from build123d import *

# Parameters (mm, degrees)
SKETCH1_W                  = 210
SKETCH1_H                  = 20
SKETCH2_R                  = 170.296824317
BOSS_EXTRUDE1_DEPTH        = 170
BOSS_EXTRUDE1_TAPER        = 16.950103548
F_8_4_8_4_DIAMETER_HOLE1_D = 8.4
F_8_4_8_4_DIAMETER_HOLE2_D = 8.4
FILLET1_R                  = 2
FILLET2_R                  = 5
FILLET3_R                  = 22
FILLET4_R                  = 25


with BuildPart() as part:
    # Sketch1 → Revolve1 (revolve)
    with BuildSketch(Plane.XZ, mode=Mode.PRIVATE) as revolve1_sk:
        with Locations((105, 10)):
            Rectangle(SKETCH1_W, SKETCH1_H)
    revolve(revolve1_sk.sketch.rotate(Axis((0, 0, 20), (0, 0, -1)), 180), axis=Axis((0, 0, 20), (0, 0, -1)))

    # Sketch2 → Boss-Extrude1 (add)
    with BuildSketch(Plane.XY.offset(20)):
        Circle(SKETCH2_R)
    extrude(amount=BOSS_EXTRUDE1_DEPTH, taper=BOSS_EXTRUDE1_TAPER)

    # Sketch3 → Cut-Revolve1 (revolve, cut)
    with BuildSketch(Plane(origin=(0, 0, 0), x_dir=(1, 0, 0), z_dir=(0, 1, 0))):
        Polygon((155.484121585, 0), (0, 0), (0, -190), (50, -190), (50, -170), (103.671746464, -170), align=None)
    revolve(axis=Axis((0, 0, 0), (0, 0, 1)), mode=Mode.SUBTRACT)

    # Ø8.4 (8.4) Diameter Hole1 (through all)
    with Locations(Plane.XY.offset(20)):
        with Locations((0, 195), (97.5, 168.874953738), (168.874953738, 97.5), (195, 0), (168.874953738, -97.5), (97.5, -168.874953738), (0, -195), (-97.5, -168.874953738), (-168.874953738, -97.5), (-195, 0), (-168.874953738, 97.5), (-97.5, 168.874953738)):
            Hole(F_8_4_8_4_DIAMETER_HOLE1_D / 2)

    # Ø8.4 (8.4) Diameter Hole2 (through all)
    with Locations(Plane(origin=(0, 0, 170), x_dir=(-1, 0, 0), z_dir=(0, 0, -1))):
        with Locations((0, 76.095238095), (38.047619048, 65.900409298), (65.900409298, 38.047619048), (76.095238095, 0), (65.900409298, -38.047619048), (38.047619048, -65.900409298), (0, -76.095238095), (-38.047619048, -65.900409298), (-65.900409298, -38.047619048), (-76.095238095, 0), (-65.900409298, 38.047619048), (-38.047619048, 65.900409298)):
            Hole(F_8_4_8_4_DIAMETER_HOLE2_D / 2)

    # Fillet1
    fillet1_edges = [part.edges().sort_by_distance(p)[0] for p in [
        (-103.671746464, 0, 170),
    ]]
    fillet(fillet1_edges, radius=FILLET1_R)

    # Fillet2
    fillet2_edges = [part.edges().sort_by_distance(p)[0] for p in [
        (-170.296824317, 0, 20),
    ]]
    fillet(fillet2_edges, radius=FILLET2_R)

    # Fillet3
    fillet3_edges = [part.edges().sort_by_distance(p)[0] for p in [
        (-118.484449196, 0, 190),
    ]]
    fillet(fillet3_edges, radius=FILLET3_R)

    # Fillet4
    fillet4_edges = [part.edges().sort_by_distance(p)[0] for p in [
        (-155.484121585, 0, 0),
    ]]
    fillet(fillet4_edges, radius=FILLET4_R)


solid = part.part
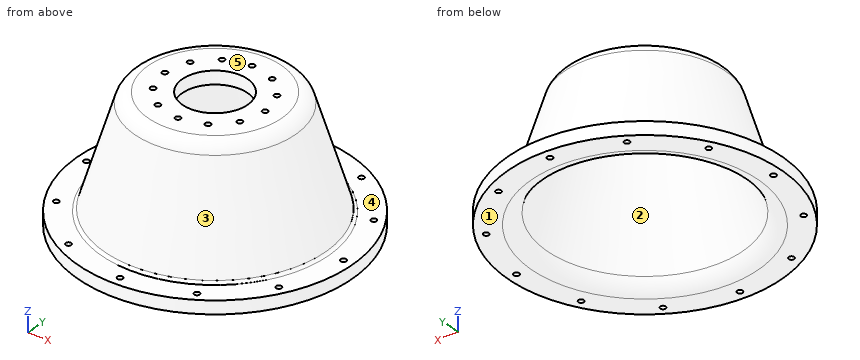
The model under review builds one solid part; all positions refer to its coordinate system, in mm. Face numbers are marked on the shaded views. A direction names the side the tool comes from. Give positions to 0.01 mm unless a question says otherwise; leave off trailing zeros. Order: outer loops, then holes, each group sorted by start corner. A loop starts at its lowest first (then second) coordinate and runs counter-clockwise, first axis right, second up. Notation, with made-up numbers: M -7.75,4 L 0.25,4 A19 ccw 0.25,10 Z; hole C -27,-14 d1. An arc over 180 degrees is marked long. One line per question, with ' | ' between items. Start each with the question number.
1) Consider section A-A, the plane z = 123.5. Give the boundary of the cut face in (x, y).
2) Wall thickness on L1, parallel to Z at x = -49, y = -70; L2, parallel to Y at x = 0, z = 178.75; L3, parallel to Y at x = -97.5, z = 10.75: over which ranges is each line inside the solid? List them lowest first. Write a range as from..to.
3) Mouldability with a two-part tool opening along Y and no side actions: class the marked faces 1, 2 and 3 as pulls with the +Y half, pulls with the -Y half, needs draft (parallel to the pull), parting line crosses it, or undercut.
4) For the marked faces 4 and 5, list the 3-axis set-ups (+Z, -Z, +X, -X, +Y, -Y) from which the entire face can be reached by the end or side of a thin tool; tool diameter is ignored.
5) Consider section B-B, the plane y = 184. Give the boundary of the cut face in (x, z), then the cut area to 3 significant figures.
6) Consider section C-C, the plane z = 75.5. Give the boundary of the cut face in (x, y), then the cut area to 3 significant figures.
7) Clearance check with flat-ended pins moving along their axes: P1, Ø8, axis at x = -113.5, z = 52, coming from the +Y side; P2, Ø9.5, axis at x = 0, y = -195, coming from the +Z side; P3, Ø11, axis at x = -38.05, y = -65.9, coming from the -Z side; P4, Ø11, axis at x = -65.9, y = -38.05, coming from the +Z side. State where each tip first meets the part, or that it passes through.
Found:
1) outline: C 0,0 d277.5; hole C 0,0 d235.69
2) L1: z = 170..190 | L2: y = -121.39..-80.3, -71.9..-50, 50..71.9, 80.3..121.39 | L3: y = -185.99..-173.07, -164.67..-118.5, 118.5..164.67, 173.07..185.99
3) face 1: needs draft | face 2: undercut | face 3: parting line crosses it
4) face 4: +Z | face 5: +Z, +X, -X, +Y, -Y
5) outline: M -101.21,0 L 101.21,0 L 101.21,20 L -101.21,20 Z | area: 4,050 mm²
6) outline: C 0,0 d306.76; hole C 0,0 d264.95 | area: 18,800 mm²
7) P1: stops at y = 117.76 | P2: stops at z = 20 | P3: stops at z = 170 | P4: stops at z = 190
